CAD build for the part. Positions are in the model's coordinates, mm. A direction names the side the tool comes from. Coordinates: 2 decimals unless noted, no trailing zeros. Write each loop counter-clockwise with the first axis right and the second up, starting at its lowest first coordinate (ties: lowest second). Pieces come first, ordered by that corner, then holes. Notation, with made-up numbers: M 48,-4.75 L 102,-4.75 A21 cw 102,3.25 Z; hole C -16.5,40 d11. An arc over 180 degrees is marked long. Answer as CSV lines item,"result". Start each with the question number.
```python
from build123d import *

# Parameters (mm, degrees)
SKETCH_1_R          = 22.5
SKETCH_1_R_2        = 15
EXTRUDE_1_DEPTH     = 64
SKETCH_2_R          = 37
SKETCH_2_R_2        = 22.5
EXTRUDE_2_DEPTH     = 10
SKETCH_3_R          = 5.5
CUT_EXTRUDE_1_DEPTH = 6.6
SKETCH_4_R          = 3.3
CUT_EXTRUDE_2_DEPTH = 65


with BuildPart() as part:
    # 草图1 → 凸台-拉伸1 (new body)
    with BuildSketch(Plane(origin=(0, 0, 0), x_dir=(1, 0, 0), z_dir=(0, 1, 0))):
        Circle(SKETCH_1_R)
        Circle(SKETCH_1_R_2, mode=Mode.SUBTRACT)
    extrude(amount=EXTRUDE_1_DEPTH)

    # 草图2 → 凸台-拉伸2 (add)
    with BuildSketch(Plane(origin=(0, 64, 0), x_dir=(1, 0, 0), z_dir=(0, 1, 0))):
        Circle(SKETCH_2_R)
        Circle(SKETCH_2_R_2, mode=Mode.SUBTRACT)
    extrude(amount=-EXTRUDE_2_DEPTH)

    # 草图3 → 切除-拉伸1 (cut)
    with BuildSketch(Plane(origin=(0, 64, 0), x_dir=(1, 0, 0), z_dir=(0, 1, 0))):
        with Locations((0, 30)):
            Circle(SKETCH_3_R)
        with Locations((30, 0)):
            Circle(SKETCH_3_R)
        with Locations((0, -30)):
            Circle(SKETCH_3_R)
        with Locations((-30, 0)):
            Circle(SKETCH_3_R)
    extrude(amount=-CUT_EXTRUDE_1_DEPTH, mode=Mode.SUBTRACT)

    # 草图4 → 切除-拉伸2 (cut, through all)
    with BuildSketch(Plane(origin=(0, 64, 0), x_dir=(1, 0, 0), z_dir=(0, 1, 0))):
        with Locations((0, 30)):
            Circle(SKETCH_4_R)
        with Locations((30, 0)):
            Circle(SKETCH_4_R)
        with Locations((0, -30)):
            Circle(SKETCH_4_R)
        with Locations((-30, 0)):
            Circle(SKETCH_4_R)
    extrude(amount=-CUT_EXTRUDE_2_DEPTH, mode=Mode.SUBTRACT)


solid = part.part
```
1) Pin check, flat tips, straight feed: P1, Ø10, axis at x = -11.5, y = 35, coming from the -Z side; P2, Ø5, axis at y = 16.5, z = -14, coming from the -X side; P3, Ø22, axis at x = 1.5, z = -6, coming from the -Y side; P4, Ø10, axis at x = 0, z = 30, coming from the +Y side. Stop position of each tip, or through.
2) Two-plate mould, pull along Z, no slides. Class faces 1 (the cylindrical face through (-8.02, 59.07, 36.12)), 2 (the flat face through (15, 0, 5)), 3 (the cylindrical face through (-26.95, 55.72, 1.26)): pulls with the +Z half, pulls with the -Z half, needs draft (parallel to the pull), parting line crosses it, or undercut.
3) Band-saw the part on A-A, the plane x = 0. List the corners of the cut face in (y, z).
4) Band-saw the part on D-D, the plane z = 29. List the corners of the cut face in (x, y), plus the area to 3 significant figures.
5) Band-saw the part on C-C, the plane y = 56. List the corners of the cut face in (x, z), plus the area to 3 significant figures.
6) Band-saw the part on B-B, the plane z = 0. List the corners of the cut face in (x, y).
7) Probe L1, parallel to Z at x = 0, y = 60.5; L2, parallel to X at y = 55.7, z = 0. List the from-to ranges inside material, lowest first. Write a range as [from, to].
8) Tool access for faces 4 (the cylindrical face through (-14.985, 31.552, -0.66)), 5 (the cylindrical face through (-0.716, 60.746, -35.453)), 6 (the flat face through (16, 54, -17)): list every direction of +Z, -Z, +X, -X, +Y, -Y with a clear straight run to the whole face (end or side of a thin tool).
Result sheet:
1,P1,"stops at z = -21.54"
1,P2,"stops at x = -19.34"
1,P3,"stops at y = 0"
1,P4,"stops at y = 57.4"
2,face 1,"parting line crosses it"
2,face 2,"needs draft"
2,face 3,"undercut"
3,outline,"M 0,-22.5 L 54,-22.5 L 54,-26.7 L 57.4,-26.7 L 57.4,-24.5 L 64,-24.5 L 64,-15 L 0,-15 Z; M 0,15 L 64,15 L 64,24.5 L 57.4,24.5 L 57.4,26.7 L 54,26.7 L 54,22.5 L 0,22.5 Z; M 54,-37 L 64,-37 L 64,-35.5 L 57.4,-35.5 L 57.4,-33.3 L 54,-33.3 Z; M 54,33.3 L 57.4,33.3 L 57.4,35.5 L 64,35.5 L 64,37 L 54,37 Z"
4,outline,"M -22.98,54 L -3.14,54 L -3.14,57.4 L -5.41,57.4 L -5.41,64 L -22.98,64 Z; M 3.14,54 L 22.98,54 L 22.98,64 L 5.41,64 L 5.41,57.4 L 3.14,57.4 Z"
4,area,"367 mm²"
5,outline,"C 0,0 d74; hole C -30,0 d6.6; hole C 0,0 d30; hole C 0,-30 d6.6; hole C 0,30 d6.6; hole C 30,0 d6.6"
5,area,"3,460 mm²"
6,outline,"M -37,54 L -33.3,54 L -33.3,57.4 L -35.5,57.4 L -35.5,64 L -37,64 Z; M -26.7,54 L -22.5,54 L -22.5,0 L -15,0 L -15,64 L -24.5,64 L -24.5,57.4 L -26.7,57.4 Z; M 15,0 L 22.5,0 L 22.5,54 L 26.7,54 L 26.7,57.4 L 24.5,57.4 L 24.5,64 L 15,64 Z; M 33.3,54 L 37,54 L 37,64 L 35.5,64 L 35.5,57.4 L 33.3,57.4 Z"
7,L1,"z = [-37, -35.5], [-24.5, -15], [15, 24.5], [35.5, 37]"
7,L2,"x = [-37, -33.3], [-26.7, -15], [15, 26.7], [33.3, 37]"
8,face 4,"+Y, -Y"
8,face 5,"+Y"
8,face 6,"-Y"
